from build123d import *


with BuildPart() as part:
    # Sketch1 → Revolve1 (revolve)
    with BuildSketch(Plane.XY):
        with BuildLine():
            Line((299.869822457, 19.969981452), (299.869822457, 581.9306305))
            add(Edge.make_bspline(
                [(260.243694036, 580.74911208), (263.082956961, 581.563236016), (266.059385675, 581.972800203), (269, 582.009104084), (279.289376505, 582.136133423), (289.579854883, 582.084453334), (299.869822457, 581.9306305)],
                knots=[1.210890247, 1.210890247, 1.210890247, 1.210890247, 2, 2, 2, 2.440961889, 2.440961889, 2.440961889, 2.440961889], degree=3))
            ThreePointArc((260.243694036, 580.74911208), (255.013666059, 577.154654049), (253, 571.136475738))
            Line((253, 571.136475738), (253, 513))
            add(Edge.make_bspline(
                [(224.604387653, 471.772395411), (231.364357938, 479.199956822), (238.40494302, 486.462792022), (245, 494), (246.09750768, 495.254294491), (247.381015539, 496.452538849), (248, 498), (248.753027097, 499.882567742), (248.575161437, 502.017420038), (249, 504), (250.83185132, 512.548639496), (248.636070132, 510.818035066), (253, 513)],
                knots=[1.073552287, 1.073552287, 1.073552287, 1.073552287, 2, 2, 2, 3, 3, 3, 4, 4, 4, 5, 5, 5, 5], degree=3))
            ThreePointArc((224.604387653, 471.772395411), (222.673797036, 468.650094884), (222, 465.041502601))
            Line((222, 465.041502601), (222, 42.919041115))
            ThreePointArc((222, 42.919041115), (222.037005327, 42.059542919), (222.14774743, 41.206405924))
            add(Edge.make_bspline(
                [(227.708226393, 27.19266873), (223.001482513, 30.417198271), (223.012565993, 36.231376239), (222.14774743, 41.206405924)],
                knots=[8.018855033, 8.018855033, 8.018855033, 8.018855033, 8.950003244, 8.950003244, 8.950003244, 8.950003244], degree=3))
            add(Edge.make_bspline(
                [(299.869822457, 19.969981452), (245.269197516, 19.906383893), (227.708226393, 27.19266873)],
                knots=[0, 0, 0, 0.455690214, 0.455690214, 0.455690214], degree=2))
        make_face()
    revolve(axis=Axis((299.869822457, 19.969981452, 0), (0, 1, 0)))


solid = part.part
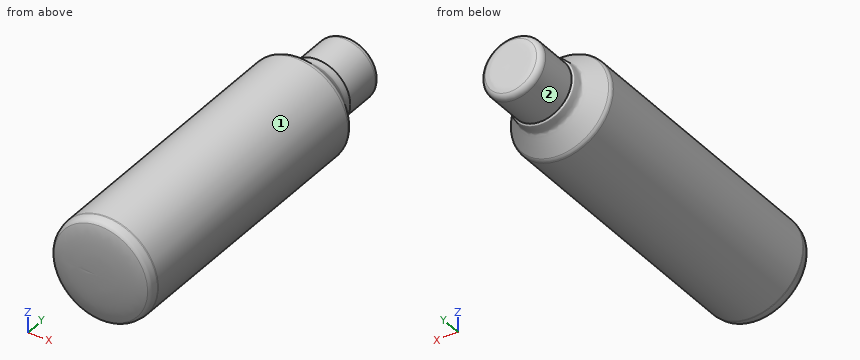
The listing builds one solid part. Answer for the finished solid, in the listing's coordinates (mm). Face numbers are marked on the shaded views. A direction names the side the tool comes from. Give positions to 0.01 mm unless a question says otherwise; leave off trailing zeros. Loops run counter-clockwise (first coordinate to the right, second up) from the corner with the lowest first, then second, coordinate; pieces in that order, holes last. Notation, with made-up numbers: (0, -32) - (14, -32) arc R32 ccw to (14, -6) - close; hole circle Ø2 at (18.25, -34). An arc over 180 degrees is marked (long way). Write each question's results on one line, items separated by ' | '.
1. Flat-ended cylindrical pins translate along their axes: P1, Ø10, axis at x = 249, y = 113, coming from the -Z side; P2, Ø10, axis at x = 336.5, y = 212, coming from the +Z side; P3, Ø8, axis at x = 317, y = 507.5, coming from the +Z side. Find the tip coordinate at first contact, or state that the pin passes through.
Resolved:
P1: stops at z = -62.93 | P2: stops at z = 71.16 | P3: stops at z = 48.69
2. Which of the six approach directions +Z, -Z, +X, -X, +Y, -Y give full straight-line access (tool end or side, diameter ignored) to the marked faces 1 and 2?
Resolved:
face 1: +Y, -Y | face 2: +Y
3. Consider probe 1 along X at (y, z) = (72, -2); probe 2 along X at (y, z) = (392, 19.5); probe 3 along Y at (x, z) = (297.5, -13.5). Determine where each line is inside the solid, lowest interval first. Write a range as from..to.
Resolved:
probe 1: x = 222.03..377.71 | probe 2: x = 224.48..375.26 | probe 3: y = 20.08..582.07
4. Find section A-A, the plane y = 528. Write down the section's boundary in (x, z), then the cut area to 3 significant figures.
Resolved:
outline: circle Ø93.74 at (299.87, 0) | area: 6,900 mm^2
5. Find section B-B, the plane y = 175.5. Write down the section's boundary in (x, z), then the cut area to 3 significant figures.
Resolved:
outline: circle Ø155.74 at (299.87, 0) | area: 19,000 mm^2
